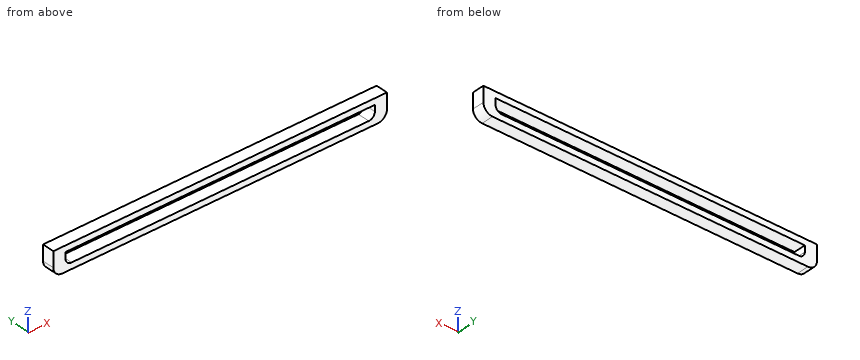
from build123d import *

# Parameters (mm, degrees)
BOX001_W     = 51
BOX001_H     = 2
BOX001_DEPTH = 2
BOX_W        = 55
BOX_H        = 2
BOX_DEPTH    = 4
FILLET_R     = 1.5
FILLET001_R  = 1
FILLET002_R  = 1


with BuildPart() as cube001:
    # Box001 → Box001 (new body)
    with BuildSketch(Plane(origin=(2, 0, 1), x_dir=(1, 0, 0), z_dir=(0, 0, 1))):
        with Locations((25.5, 1)):
            Rectangle(BOX001_W, BOX001_H)
    extrude(amount=BOX001_DEPTH)


with BuildPart() as fillet002:
    # Box → Box (new body)
    with BuildSketch(Plane.XY):
        with Locations((27.5, 1)):
            Rectangle(BOX_W, BOX_H)
    extrude(amount=BOX_DEPTH)

    # Cut: cut Cube001
    add(cube001.part, mode=Mode.SUBTRACT)

    # Fillet
    fillet_edges = [fillet002.edges().sort_by_distance(p)[0] for p in [
        (0, 1, 0),
        (55, 1, 0),
    ]]
    fillet(fillet_edges, radius=FILLET_R)

    # Fillet001
    fillet001_edges = [fillet002.edges().sort_by_distance(p)[0] for p in [
        (2, 1, 1),
    ]]
    fillet(fillet001_edges, radius=FILLET001_R)

    # Fillet002
    fillet002_edges = [fillet002.edges().sort_by_distance(p)[0] for p in [
        (53, 1, 1),
    ]]
    fillet(fillet002_edges, radius=FILLET002_R)


solid = fillet002.part
Build history of the part. All positions in model axes, mm. Round coordinates to 2 decimals unless told otherwise and drop trailing zeros. Write each loop counter-clockwise with the first axis right and the second up, starting at its lowest first coordinate (ties: lowest second). Pieces come first, ordered by that corner, then holes. Notation, with made-up numbers: (-17, 84) -> (41, 84) arc R21 ccw to (41, 98) -> close; hole circle Ø7 at (-36.75, 46). An arc over 180 degrees is marked (long way). Use one line per item in the form item = value.
Q1. Band-saw the part on A-A, the plane y = 0.75. Write the cut outline in (x, z).
Conclusion:
outline = (0, 1.5) arc R1.5 ccw to (1.5, 0) -> (53.5, 0) arc R1.5 ccw to (55, 1.5) -> (55, 4) -> (0, 4) -> close; hole (2, 2) arc R1 ccw to (3, 1) -> (52, 1) arc R1 ccw to (53, 2) -> (53, 3) -> (2, 3) -> close
Q2. Drill centre lines: L1, parallel to Z at x = 43, y = 0.8; L2, parallel to X at y = 1.3, z = 2.2; L3, parallel to X at y = 1.95, z = 1.15. Where is each one in solid material? Low to high.
Conclusion:
L1 = 0 to 1, 3 to 4
L2 = 0 to 2, 53 to 55
L3 = 0.04 to 2.47, 52.53 to 54.96
Q3. Band-saw the part on B-B, the plane x = 10.5. Write the cut outline in (y, z).
Conclusion:
outline = (0, 0) -> (2, 0) -> (2, 1) -> (0, 1) -> close; (0, 3) -> (2, 3) -> (2, 4) -> (0, 4) -> close
